from build123d import *

# Parameters (mm, degrees)
SKETCH1_W           = 25
SKETCH1_H           = 18
SKETCH1_W_2         = 19
SKETCH1_H_2         = 13
BOSS_EXTRUDE1_DEPTH = 5
SKETCH2_R           = 1.5
BOSS_EXTRUDE2_DEPTH = 5
FILLET1_R           = 5


with BuildPart() as part:
    # Sketch1 → Boss-Extrude1 (new body)
    with BuildSketch(Plane.XY):
        Rectangle(SKETCH1_W, SKETCH1_H)
        Rectangle(SKETCH1_W_2, SKETCH1_H_2, mode=Mode.SUBTRACT)
    extrude(amount=BOSS_EXTRUDE1_DEPTH)

    # Sketch2 → Boss-Extrude2 (add)
    # profile 1 of 2: a face of its own
    with BuildSketch(Plane(origin=(0, 0, 0), x_dir=(-1, 0, 0), z_dir=(0, 0, -1))):
        with BuildLine():
            Line((-17.5, 3), (-12.5, 3))
            Line((-12.5, 3), (-12.5, -3))
            Line((-12.5, -3), (-17.5, -3))
            ThreePointArc((-17.5, -3), (-20.5, 0), (-17.5, 3))
        make_face()
        with Locations((-17.5, 0)):
            Circle(SKETCH2_R, mode=Mode.SUBTRACT)
    # profile 2 of 2: a face of its own
    with BuildSketch(Plane(origin=(0, 0, 0), x_dir=(-1, 0, 0), z_dir=(0, 0, -1))):
        with BuildLine():
            Line((17.5, 3), (12.5, 3))
            Line((12.5, 3), (12.5, -3))
            Line((12.5, -3), (17.5, -3))
            ThreePointArc((17.5, -3), (20.5, 0), (17.5, 3))
        make_face()
        with Locations(Location((17.5, 0, 0), (0, 0, 180))):
            Circle(SKETCH2_R, mode=Mode.SUBTRACT)
    extrude(amount=-BOSS_EXTRUDE2_DEPTH)

    # Fillet1
    fillet1_edges = [part.edges().sort_by_distance(p)[0] for p in [
        (12.5, -3, 2.5),
        (-12.5, -3, 2.5),
        (-12.5, 3, 2.5),
        (12.5, 3, 2.5),
    ]]
    fillet(fillet1_edges, radius=FILLET1_R - 0.0001)  # a hair under: the kernel refuses the full size


solid = part.part
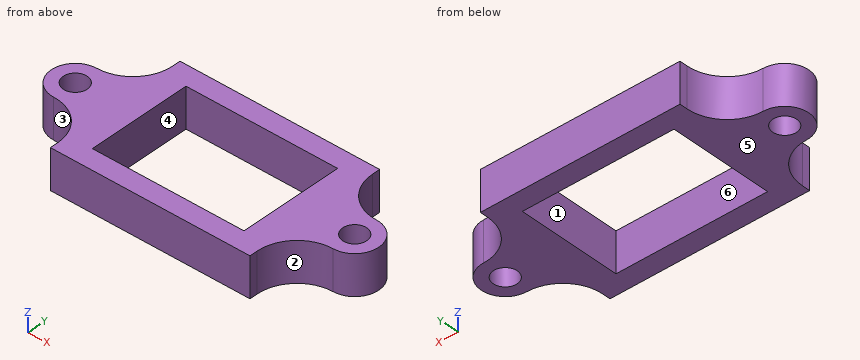
Model file for the job. Use its own axes, mm. Face numbers are marked on the shaded views. A direction names the side the tool comes from. Round coordinates to 2 decimals unless told otherwise and drop trailing zeros. Loops run counter-clockwise (first coordinate to the right, second up) from the corner with the lowest first, then second, coordinate; pieces in that order, holes last. Notation, with made-up numbers: (19.25, 35.25) -> (45.25, 35.25) arc R22 ccw to (45.25, 74.25) -> close; hole circle Ø4 at (4.5, -2). An arc over 180 degrees is marked (long way). Answer as CSV lines item,"result". Start each with the question number.
1) Slice it at A-A (x = -0.5). List the corners of the cut face in (y, z).
2) Slice it at D-D (y = 0). List the corners of the cut face in (x, z), plus the area to 3 significant figures.
3) Tool access for the marked faces 1 and 2: list every direction of +Z, -Z, +X, -X, +Y, -Y with a clear straight run to the whole face (end or side of a thin tool).
4) Mould opens along Y. For the marked faces 3, 4, 5 and 6 say: +Y half, -Y half, draft (parallel to the pull), parting line (faces both ways), or undercut.
5) Pin check, flat tips, straight feed: P1, Ø0.5, axis at y = 8.5, z = 3.5, coming from the +X side; P2, Ø0.5, axis at y = 8.5, z = 2, coming from the -X side; P3, Ø2, axis at y = 6, z = 3.5, coming from the -X side. Stop position of each tip, or through.
6) Slice it at C-C (z = 2.55). State how many separate pieces and enclosed holes the cut face has, plus the area to 3 significant figures.
7) Slice it at B-B (y = 6). List the corners of the cut face in (x, z).
8) Probe line 1 along Y through (x, z) = (-1.5, 3.4); line 2 along X through (y, z) = (0.5, 0.3); line 3 along X through (y, z) = (1.25, 1.5). List the from-to ranges inside material, lowest first.
Filled in:
1,outline,"(-9, 0) -> (-6.5, 0) -> (-6.5, 5) -> (-9, 5) -> close; (6.5, 0) -> (9, 0) -> (9, 5) -> (6.5, 5) -> close"
2,outline,"(-20.5, 0) -> (-19, 0) -> (-19, 5) -> (-20.5, 5) -> close; (-16, 0) -> (-9.5, 0) -> (-9.5, 5) -> (-16, 5) -> close; (9.5, 0) -> (16, 0) -> (16, 5) -> (9.5, 5) -> close; (19, 0) -> (20.5, 0) -> (20.5, 5) -> (19, 5) -> close"
2,area,"80.0 mm2"
3,face 1,"+Z, -Z"
3,face 2,"+Z, -Z, +X, -Y"
4,face 3,"-Y half"
4,face 4,"undercut"
4,face 5,"draft"
4,face 6,"undercut"
5,P1,"stops at x = 12.5"
5,P2,"stops at x = -12.5"
5,P3,"stops at x = -13.5"
6,separate pieces,"1"
6,enclosed holes,"3"
6,area,"299 mm2"
7,outline,"(-12.92, 0) -> (-9.5, 0) -> (-9.5, 5) -> (-12.92, 5) -> close; (9.5, 0) -> (12.92, 0) -> (12.92, 5) -> (9.5, 5) -> close"
8,line 1,"y = -9 to -6.5, 6.5 to 9"
8,line 2,"x = -20.46 to -18.91, -16.09 to -9.5, 9.5 to 16.09, 18.91 to 20.46"
8,line 3,"x = -20.23 to -18.33, -16.67 to -9.5, 9.5 to 16.67, 18.33 to 20.23"
